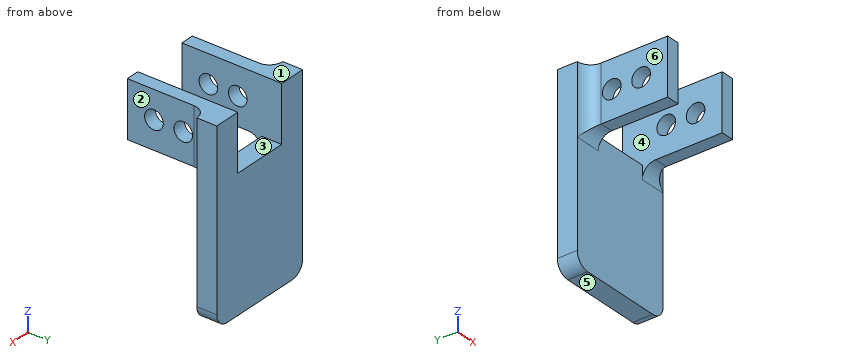
from build123d import *

# Parameters (mm, degrees)
BOSS_EXTRUDE1_DEPTH = 7.5
SKETCH2_W           = 5
SKETCH2_H           = 21
BOSS_EXTRUDE2_DEPTH = 30
SKETCH3_R           = 3.5
CUT_EXTRUDE1_DEPTH  = 79.238417673
FILLET1_R           = 5


with BuildPart() as part:
    # Sketch1 → Boss-Extrude1 (new body)
    with BuildSketch(Plane(origin=(0, 0, 0), x_dir=(1, 0, 0), z_dir=(0, 1, 0))):
        Polygon((-20.5, -10.5), (-10.5, -10.5), (-10.5, 10.5), (10.5, 10.5), (10.5, -10.5), (20.5, -10.5), (20.5, 59.5), (-20.5, 59.5), align=None)
    extrude(amount=BOSS_EXTRUDE1_DEPTH)

    # Sketch2 → Boss-Extrude2 (add)
    with BuildSketch(Plane.XZ):
        with Locations((-13, 0)):
            Rectangle(SKETCH2_W, SKETCH2_H)
        with Locations((13, 0)):
            Rectangle(SKETCH2_W, SKETCH2_H)
    extrude(amount=BOSS_EXTRUDE2_DEPTH)

    # Sketch3 → Cut-Extrude1 (cut, through all)
    with BuildSketch(Plane(origin=(20.5, 0, 0), x_dir=(0, 0, -1), z_dir=(1, 0, 0))):
        with Locations((0, -9)):
            Circle(SKETCH3_R)
        with Locations((0, -20)):
            Circle(SKETCH3_R)
    extrude(amount=-CUT_EXTRUDE1_DEPTH, mode=Mode.SUBTRACT)

    # Fillet1
    fillet1_edges = [part.edges().sort_by_distance(p)[0] for p in [
        (-13, 0, -10.5),
        (13, 0, -10.5),
        (-15.5, 0, 0),
        (15.5, 0, 0),
    ]]
    fillet(fillet1_edges, radius=FILLET1_R - 0.0001)  # a hair under: the kernel refuses the full size
    fillet1_2_edges = [part.edges().sort_by_distance(p)[0] for p in [
        (-20.5, 3.75, -59.5),
        (20.5, 3.75, -59.5),
    ]]
    fillet(fillet1_2_edges, radius=FILLET1_R)


solid = part.part
Could you check a few things on this model? Use its own coordinates, in mm. Face numbers are marked on the shaded views. A direction names the side the tool comes from. Give positions to 0.01 mm unless a question says otherwise; leave off trailing zeros. Order: outer loops, then holes, each group sorted by start corner. A loop starts at its lowest first (then second) coordinate and runs counter-clockwise, first axis right, second up. Notation, with made-up numbers: (48.25, -32) -> (80.25, -32) arc R20 ccw to (80.25, -17) -> close; hole circle Ø5 at (29, 81). An arc over 180 degrees is marked (long way). Answer in a Markdown table with one row per item. Add a question column.
Item 1: For the marked faces 1, 2 and 3, which set-ups out of +Z, -Z, +X, -X, +Y, -Y let a thin tool reach every point of the face, with its end or its side?
Item 2: Imagine slicing it at C-C (y = -25.5). List the corners of the cut face in (x, z) for me, and give its area (3 significant figures).
Item 3: Please list where these lines run through material, in increasing order: probe 1 along Y at (x, z) = (12.7, 0); probe 2 along X at (y, z) = (3, 1.5); probe 3 along Y at (x, z) = (-3.5, -50).
Item 4: We'd pull the mould along X, two halves only. Please class the marked faces 4, 5 and 6: pulls with the +X half, pulls with the -X half, needs draft (parallel to the pull), parting line crosses it, or undercut.
Item 5: Imagine slicing it at B-B (z = 0). Count the separate pieces of the cut face and the enclosed holes in it, and give its area (3 significant figures).
Item 6: Imagine slicing it at D-D (x = 2). List the corners of the cut face in (y, z) for me.
Item 7: I'm going to push flat-ended pins straight in: P1, Ø10.5, axis at y = -20.5, z = -0.5, coming from the -X side; P2, Ø13, axis at y = -10, z = 0.5, coming from the -X side; P3, Ø9, axis at y = -9, z = 0, coming from the +X side; P4, Ø4, axis at y = -9, z = 0, coming from the +X side. Where does each tip first touch, or does it pass through?
Item 8: Imagine slicing it at A-A (y = -9). List the corners of the cut face in (x, z) for me.
Result:
| question | item | result |
|---|---|---|
| 1 | face 1 | +Z, +X, -X, +Y, -Y |
| 1 | face 2 | +Z, -Z, +X, -Y |
| 1 | face 3 | +Z, +Y, -Y |
| 2 | outline | (-15.5, -10.5) -> (-10.5, -10.5) -> (-10.5, 10.5) -> (-15.5, 10.5) -> close; (10.5, -10.5) -> (15.5, -10.5) -> (15.5, 10.5) -> (10.5, 10.5) -> close |
| 2 | area | 210 mm2 |
| 3 | probe 1 | -30 to -23.5, -16.5 to -12.5, -5.5 to 7.5 |
| 3 | probe 2 | -20.5 to -10.5, 10.5 to 20.5 |
| 3 | probe 3 | 0 to 7.5 |
| 4 | face 4 | undercut |
| 4 | face 5 | needs draft |
| 4 | face 6 | pulls with the -X half |
| 5 | separate pieces | 6 |
| 5 | enclosed holes | 0 |
| 5 | area | 321 mm2 |
| 6 | outline | (0, -59.5) -> (7.5, -59.5) -> (7.5, -10.5) -> (0, -10.5) -> close |
| 7 | P1 | x = -15.5 |
| 7 | P2 | x = -15.73 |
| 7 | P3 | x = 15.53 |
| 7 | P4 | through |
| 8 | outline | (-15.5, -10.5) -> (-10.5, -10.5) -> (-10.5, -3.5) -> (-15.5, -3.5) -> close; (-15.5, 3.5) -> (-10.5, 3.5) -> (-10.5, 10.5) -> (-15.5, 10.5) -> close; (10.5, -10.5) -> (15.5, -10.5) -> (15.5, -3.5) -> (10.5, -3.5) -> close; (10.5, 3.5) -> (15.5, 3.5) -> (15.5, 10.5) -> (10.5, 10.5) -> close |
